Here's the drawing with two shaded views (mm, measured from the low corner). I have some questions. A direction names the side the tool comes from. Coordinates: 2 decimals unless noted, no trailing zeros. Write each loop counter-clockwise with the first axis right and the second up, starting at its lowest first coordinate (ties: lowest second). Pieces come first, ordered by that corner, then holes. Notation, with made-up numbers: (-12, -38) -> (3, -38) arc R10 cw to (3, -19) -> close; hole circle Ø1 at (-18, 4). An arc over 180 degrees is marked (long way). Put each result on its own line as item: value.
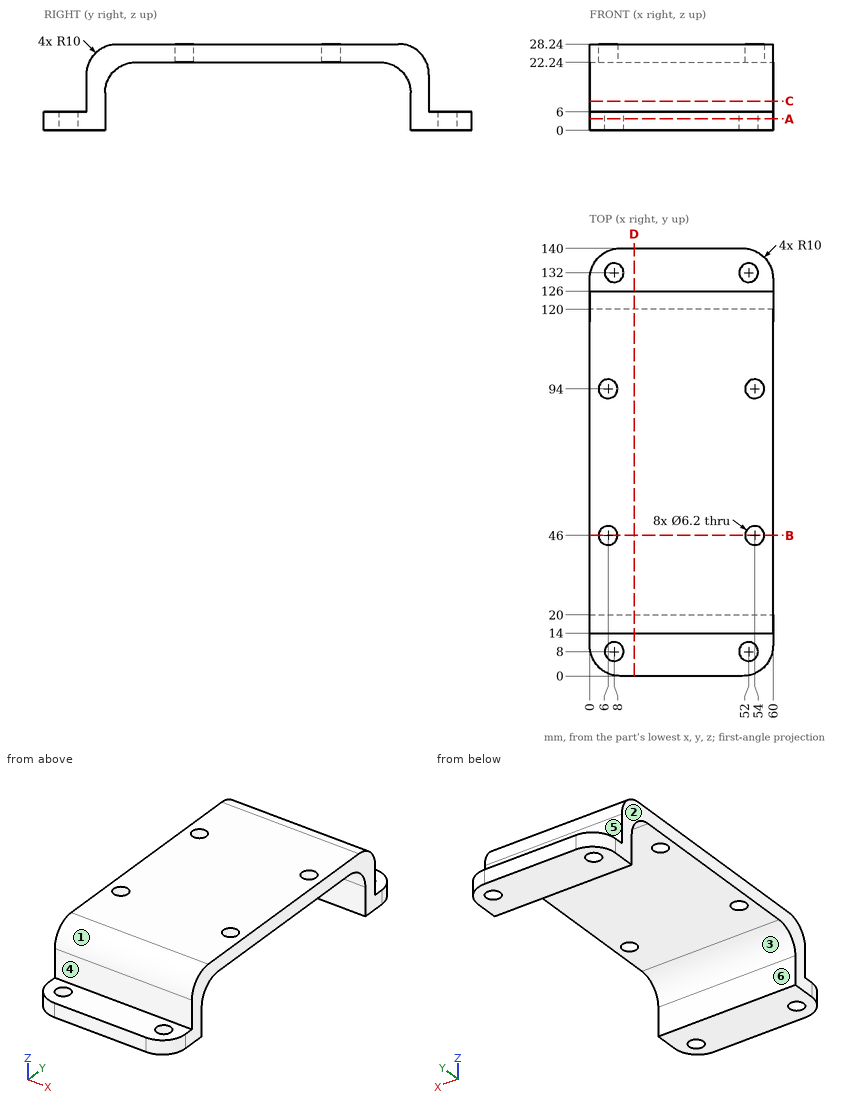
Item 1: For P1, Ø7, axis at x = 8, y = 8, coming from the +Z side; P2, Ø3.5, axis at x = 33, z = 14, coming from the -Y side; P3, Ø6, axis at x = 49, z = 12, coming from the +Y side, each with a flat end and sliding along its axis, tell me the tip position at first contact or that it passes through.
Output:
P1: stops at z = 6
P2: stops at y = 14
P3: stops at y = 126
Item 2: If we mould it in two halves opening along Y, with no side actions, what happens to the marked faces 1, 2 and 3? For each: released by +Y, released by -Y, zero draft, split by the parting line, or undercut.
Output:
face 1: released by -Y
face 2: zero draft
face 3: undercut
Item 3: Imagine slicing it at D-D on x = 14.5. Write out the boundary of the cut face in (y, z).
Output:
outline: (0, 0) -> (20, 0) -> (20, 12.24) arc R10 cw to (30, 22.24) -> (110, 22.24) arc R10 cw to (120, 12.24) -> (120, 0) -> (140, 0) -> (140, 6) -> (126, 6) -> (126, 18.24) arc R10 ccw to (116, 28.24) -> (24, 28.24) arc R10 ccw to (14, 18.24) -> (14, 6) -> (0, 6) -> close
Item 4: Which directions (+Z, -Z, +X, -X, +Y, -Y) give clear straight access to the entire face, cutting with the end or side of a thin tool? Please do the marked faces 4, 5 and 6.
Output:
face 4: +Z, +X, -X, -Y
face 5: +Z, +X, -X, +Y
face 6: -Z, +X, -X
Item 5: Imagine slicing it at C-C on z = 9.5. Write out the boundary of the cut face in (x, y), then the cut area to 3 significant figures.
Output:
outline: (0, 14) -> (60, 14) -> (60, 20) -> (0, 20) -> close; (0, 120) -> (60, 120) -> (60, 126) -> (0, 126) -> close
area: 720 mm²
Item 6: Imagine slicing it at A-A on z = 3.75. Write out the boundary of the cut face in (x, y), then the cut area to 3 significant figures.
Output:
outline: (0, 10) arc R10 ccw to (10, 0) -> (50, 0) arc R10 ccw to (60, 10) -> (60, 20) -> (0, 20) -> close; (0, 120) -> (60, 120) -> (60, 130) arc R10 ccw to (50, 140) -> (10, 140) arc R10 ccw to (0, 130) -> close; hole circle Ø6.2 at (8, 8); hole circle Ø6.2 at (8, 132); hole circle Ø6.2 at (52, 8); hole circle Ø6.2 at (52, 132)
area: 2,190 mm²
Item 7: Please list where these lines run through material, in increasing order: line 1 along X through (y, z) = (46, 25.5); line 2 along Y through (x, z) = (54, 26.4); line 3 along Y through (x, z) = (54, 25.05). Write a range as from..to.
Output:
line 1: x = 0..2.9, 9.1..50.9, 57.1..60
line 2: y = 18.22..42.9, 49.1..90.9, 97.1..121.78
line 3: y = 16.68..42.9, 49.1..90.9, 97.1..123.32
Item 8: Imagine slicing it at B-B on y = 46. Write out the boundary of the cut face in (x, z).
Output:
outline: (0, 22.24) -> (2.9, 22.24) -> (2.9, 28.24) -> (0, 28.24) -> close; (9.1, 22.24) -> (50.9, 22.24) -> (50.9, 28.24) -> (9.1, 28.24) -> close; (57.1, 22.24) -> (60, 22.24) -> (60, 28.24) -> (57.1, 28.24) -> close
